Job drawing, mm, ordinate dimensions from the low corner. One solid piece. A direction names the side the tool comes from. Round coordinates to 2 decimals unless told otherwise and drop trailing zeros. Loops run counter-clockwise (first coordinate to the right, second up) from the corner with the lowest first, then second, coordinate; pieces in that order, holes last. Notation, with made-up numbers: M -9,64.5 L 43,64.5 A12 ccw 43,75.5 Z; hole C 82,48 d1. An arc over 180 degrees is marked long. Write each question's results on one line, items separated by ' | '. Start each with the question number.
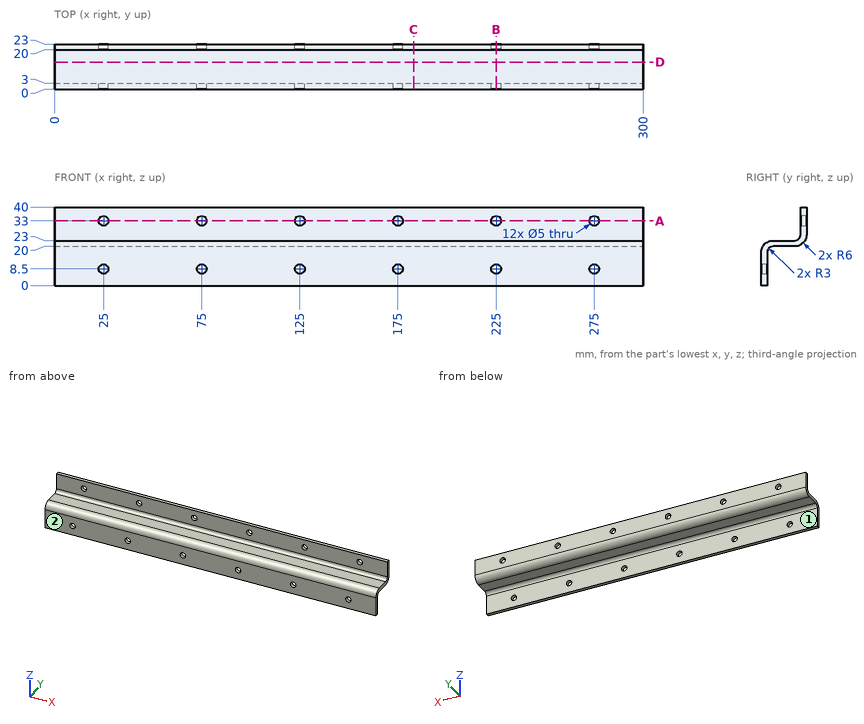
Item 1: Saw through at A-A, the plane z = 33. Give the cut face in (x, y), then the cut area to 3 significant figures.
Item 2: Saw through at C-C, the plane x = 183. Give the cut face in (y, z).
Item 3: Saw through at D-D, the plane y = 13.75. Give the cut face in (x, z).
Item 4: Drill centre lines: line 1 along Z through (x, y) = (225, 21.9); line 2 along Z through (x, y) = (162, 11.5); line 3 along Y through (x, z) = (228, 12). Where is each one in solid material? Low to high. Write a range as [from, to].
Item 5: Drop flat-ended pins along their axis: pin 1 (4 mm diameter, centred on x = 51, z = 30, fed in from -Y); pin 2 (9 mm diameter, centred on x = 133.5, y = 14, fed in from -Z); pin 3 (10 mm diameter, centred on y = 3, z = 24, fed in from -X); pin 4 (6.5 mm diameter, centred on x = 125, z = 8.5, fed in from +Y). Give the stop position or say it passes through.
Item 6: Saw through at B-B, the plane x = 225. Give the cut face in (y, z).
Item 7: Tool access for the marked faces 1 and 2: list every direction of +Z, -Z, +X, -X, +Y, -Y with a clear straight run to the whole face (end or side of a thin tool).
Working result:
1) outline: M 0,20 L 22.5,20 L 22.5,23 L 0,23 Z; M 27.5,20 L 72.5,20 L 72.5,23 L 27.5,23 Z; M 77.5,20 L 122.5,20 L 122.5,23 L 77.5,23 Z; M 127.5,20 L 172.5,20 L 172.5,23 L 127.5,23 Z; M 177.5,20 L 222.5,20 L 222.5,23 L 177.5,23 Z; M 227.5,20 L 272.5,20 L 272.5,23 L 227.5,23 Z; M 277.5,20 L 300,20 L 300,23 L 277.5,23 Z | area: 810 mm²
2) outline: M 0,0 L 3,0 L 3,17 A3 cw 6,20 L 17,20 A6 ccw 23,26 L 23,40 L 20,40 L 20,26 A3 cw 17,23 L 6,23 A6 ccw 0,17 Z
3) outline: M 0,20 L 300,20 L 300,23 L 0,23 Z
4) line 1: z = [22.54, 30.5], [35.5, 40] | line 2: z = [20, 23] | line 3: y = [0, 3]
5) pin 1: stops at y = 20 | pin 2: stops at z = 20 | pin 3: stops at x = 0 | pin 4: stops at y = 3
6) outline: M 0,0 L 3,0 L 3,6 L 0,6 Z; M 0,11 L 3,11 L 3,17 A3 cw 6,20 L 17,20 A6 ccw 23,26 L 23,30.5 L 20,30.5 L 20,26 A3 cw 17,23 L 6,23 A6 ccw 0,17 Z; M 20,35.5 L 23,35.5 L 23,40 L 20,40 Z
7) face 1: -Z, +X, -X, +Y | face 2: +Z, -Z, +X, -X, -Y
